```python
from build123d import *

# Parameters (mm, degrees)
SKETCH3_R           = 27.045923136
BOSS_EXTRUDE1_DEPTH = 5.6
SKETCH4_R           = 1.5
CUT_EXTRUDE1_DEPTH  = 6.6
BOSS_EXTRUDE3_DEPTH = 5.6
SKETCH6_R           = 4.2
BOSS_EXTRUDE4_DEPTH = 8.4
SKETCH7_W           = 5.4
SKETCH7_H           = 3.76
CUT_EXTRUDE2_DEPTH  = 6
FILLET1_R           = 4


with BuildPart() as part:
    # Sketch3 → Boss-Extrude1 (new body)
    with BuildSketch(Plane(origin=(0, 0, 0), x_dir=(0, 0, -1), z_dir=(1, 0, 0))):
        Circle(SKETCH3_R)
    extrude(amount=BOSS_EXTRUDE1_DEPTH)

    # Sketch4 → Cut-Extrude1 (cut, through all)
    with BuildSketch(Plane(origin=(5.6, 0, 0), x_dir=(0, 0, -1), z_dir=(1, 0, 0))):
        with Locations((0, 27.045923136)):
            Circle(SKETCH4_R)
        with Locations((13.522961568, 23.422456505)):
            Circle(SKETCH4_R)
        with Locations((23.422456505, 13.522961568)):
            Circle(SKETCH4_R)
        with Locations((27.045923136, 0)):
            Circle(SKETCH4_R)
        with Locations((23.422456505, -13.522961568)):
            Circle(SKETCH4_R)
        with Locations((13.522961568, -23.422456505)):
            Circle(SKETCH4_R)
        with Locations((0, -27.045923136)):
            Circle(SKETCH4_R)
        with Locations((-13.522961568, -23.422456505)):
            Circle(SKETCH4_R)
        with Locations((-23.422456505, -13.522961568)):
            Circle(SKETCH4_R)
        with Locations((-27.045923136, 0)):
            Circle(SKETCH4_R)
        with Locations((-23.422456505, 13.522961568)):
            Circle(SKETCH4_R)
        with Locations((-13.522961568, 23.422456505)):
            Circle(SKETCH4_R)
    extrude(amount=-CUT_EXTRUDE1_DEPTH, mode=Mode.SUBTRACT)

    # Sketch5 → Boss-Extrude3 (add)
    with BuildSketch(Plane(origin=(5.6, 0, 0), x_dir=(0, 0, -1), z_dir=(1, 0, 0))):
        with BuildLine():
            Line((1.499423149, 27.004327218), (4.76164368, 32.654658924))
            ThreePointArc((4.76164368, 32.654658924), (8.541028488, 31.875552268), (12.203625071, 30.660586021))
            Line((12.203625071, 30.660586021), (12.203625071, 24.136144957))
            Line((12.203625071, 24.136144957), (2.679491924, 10))
            Line((2.679491924, 10), (1.499423149, 27.004327218))
        make_face()
        with BuildLine():
            Line((22.636721809, 14.800702147), (7.320508076, 7.320508076))
            Line((7.320508076, 7.320508076), (14.800702147, 22.636721809))
            Line((14.800702147, 22.636721809), (20.451033853, 25.89894234))
            ThreePointArc((20.451033853, 25.89894234), (23.334523779, 23.334523779), (25.89894234, 20.451033853))
            Line((25.89894234, 20.451033853), (22.636721809, 14.800702147))
        make_face()
        with BuildLine():
            Line((27.004327218, 1.499423149), (10, 2.679491924))
            Line((10, 2.679491924), (24.136144957, 12.203625071))
            Line((24.136144957, 12.203625071), (30.660586021, 12.203625071))
            ThreePointArc((30.660586021, 12.203625071), (31.875552268, 8.541028488), (32.654658924, 4.76164368))
            Line((32.654658924, 4.76164368), (27.004327218, 1.499423149))
        make_face()
        with BuildLine():
            Line((24.136144957, -12.203625071), (10, -2.679491924))
            Line((10, -2.679491924), (27.004327218, -1.499423149))
            Line((27.004327218, -1.499423149), (32.654658924, -4.76164368))
            ThreePointArc((32.654658924, -4.76164368), (31.875552268, -8.541028488), (30.660586021, -12.203625071))
            Line((30.660586021, -12.203625071), (24.136144957, -12.203625071))
        make_face()
        with BuildLine():
            Line((14.800702147, -22.636721809), (7.320508076, -7.320508076))
            Line((7.320508076, -7.320508076), (22.636721809, -14.800702147))
            Line((22.636721809, -14.800702147), (25.89894234, -20.451033853))
            ThreePointArc((25.89894234, -20.451033853), (23.334523779, -23.334523779), (20.451033853, -25.89894234))
            Line((20.451033853, -25.89894234), (14.800702147, -22.636721809))
        make_face()
        with BuildLine():
            Line((1.499423149, -27.004327218), (2.679491924, -10))
            Line((2.679491924, -10), (12.203625071, -24.136144957))
            Line((12.203625071, -24.136144957), (12.203625071, -30.660586021))
            ThreePointArc((12.203625071, -30.660586021), (8.541028488, -31.875552268), (4.76164368, -32.654658924))
            Line((4.76164368, -32.654658924), (1.499423149, -27.004327218))
        make_face()
        with BuildLine():
            Line((-12.203625071, -24.136144957), (-2.679491924, -10))
            Line((-2.679491924, -10), (-1.499423149, -27.004327218))
            Line((-1.499423149, -27.004327218), (-4.76164368, -32.654658924))
            ThreePointArc((-4.76164368, -32.654658924), (-8.541028488, -31.875552268), (-12.203625071, -30.660586021))
            Line((-12.203625071, -30.660586021), (-12.203625071, -24.136144957))
        make_face()
        with BuildLine():
            Line((-22.636721809, -14.800702147), (-7.320508076, -7.320508076))
            Line((-7.320508076, -7.320508076), (-14.800702147, -22.636721809))
            Line((-14.800702147, -22.636721809), (-20.451033853, -25.89894234))
            ThreePointArc((-20.451033853, -25.89894234), (-23.334523779, -23.334523779), (-25.89894234, -20.451033853))
            Line((-25.89894234, -20.451033853), (-22.636721809, -14.800702147))
        make_face()
        with BuildLine():
            Line((-27.004327218, -1.499423149), (-10, -2.679491924))
            Line((-10, -2.679491924), (-24.136144957, -12.203625071))
            Line((-24.136144957, -12.203625071), (-30.660586021, -12.203625071))
            ThreePointArc((-30.660586021, -12.203625071), (-31.875552268, -8.541028488), (-32.654658924, -4.76164368))
            Line((-32.654658924, -4.76164368), (-27.004327218, -1.499423149))
        make_face()
        with BuildLine():
            Line((-24.136144957, 12.203625071), (-10, 2.679491924))
            Line((-10, 2.679491924), (-27.004327218, 1.499423149))
            Line((-27.004327218, 1.499423149), (-32.654658924, 4.76164368))
            ThreePointArc((-32.654658924, 4.76164368), (-31.875552268, 8.541028488), (-30.660586021, 12.203625071))
            Line((-30.660586021, 12.203625071), (-24.136144957, 12.203625071))
        make_face()
        with BuildLine():
            Line((-14.800702147, 22.636721809), (-7.320508076, 7.320508076))
            Line((-7.320508076, 7.320508076), (-22.636721809, 14.800702147))
            Line((-22.636721809, 14.800702147), (-25.89894234, 20.451033853))
            ThreePointArc((-25.89894234, 20.451033853), (-23.334523779, 23.334523779), (-20.451033853, 25.89894234))
            Line((-20.451033853, 25.89894234), (-14.800702147, 22.636721809))
        make_face()
        with BuildLine():
            Line((-1.499423149, 27.004327218), (-2.679491924, 10))
            Line((-2.679491924, 10), (-12.203625071, 24.136144957))
            Line((-12.203625071, 24.136144957), (-12.203625071, 30.660586021))
            ThreePointArc((-12.203625071, 30.660586021), (-8.541028488, 31.875552268), (-4.76164368, 32.654658924))
            Line((-4.76164368, 32.654658924), (-1.499423149, 27.004327218))
        make_face()
    extrude(amount=-BOSS_EXTRUDE3_DEPTH)

    # Sketch6 → Boss-Extrude4 (add)
    with BuildSketch(Plane(origin=(5.6, 0, 0), x_dir=(0, 0, -1), z_dir=(1, 0, 0))):
        Circle(SKETCH6_R)
    extrude(amount=BOSS_EXTRUDE4_DEPTH)

    # Sketch7 → Cut-Extrude2 (cut)
    with BuildSketch(Plane(origin=(14, 0, 0), x_dir=(0, 0, -1), z_dir=(1, 0, 0))):
        Rectangle(SKETCH7_W, SKETCH7_H)
    extrude(amount=-CUT_EXTRUDE2_DEPTH, mode=Mode.SUBTRACT)

    # Fillet1
    fillet1_edges = [part.edges().sort_by_distance(p)[0] for p in [
        (5.6, 0, 4.2),
    ]]
    fillet(fillet1_edges, radius=FILLET1_R)


solid = part.part
```
Model file for the job. Use its own axes, mm. A direction names the side the tool comes from. Coordinates: 2 decimals unless noted, no trailing zeros. Order: outer loops, then holes, each group sorted by start corner. A loop starts at its lowest first (then second) coordinate and runs counter-clockwise, first axis right, second up. Notation, with made-up numbers: (42, -25) - (98, -25) arc R35 ccw to (98, 8) - close; hole circle Ø9 at (-16.5, 9). An arc over 180 degrees is marked (long way). Return JSON: item names as keys, results as strings. Group by question number.
1) Tool access for faces 1 (the flat face through (3, 12.204, -27)), 2 (the flat face through (2.839, -24.245, 17.586)), 3 (the flat face through (2.84, 29.79, -3.11)), 4 (the flat face through (3, -12.204, 27)), 5 (the flat face through (5.6, -7, 7)): list every direction of +Z, -Z, +X, -X, +Y, -Y with a clear straight run to the whole face (end or side of a thin tool).
2) Mould opens along Y. For faces 6 (the cylindrical face through (2.839, 12.745, 22.14)), 7 (the cylindrical face through (2.839, -12.745, -22.14)), 8 (the cylindrical face through (2.839, -8.593, 31.862)), 9 (the flat face through (2.839, 24.245, -17.586)) say: released by +Y, released by -Y, zero draft, split by the parting line, or undercut.
3) Saw through at A-A, the plane x = 10.75. Write the cut outline in (y, z), plus the area to 3 significant figures.
4) Saw through at C-C, the plane y = 0. Write the cut outline in (x, z).
5) Probe line 1 (Y direction, x = 0.5, z = -27); line 2 (X direction, y = 9, z = 2.5); line 3 (X direction, y = 6, z = -4.5). List the from-to ranges inside material, lowest first. Write a range as from..to.
6) Flat gauge pins, fed straight in: P1, Ø1, axis at x = 11.5, z = 0, coming from the +Y side; P2, Ø1, axis at y = -15, z = 19, coming from the +X side; P3, Ø3, axis at x = 3.5, z = 27, coming from the +Y side; P4, Ø8, axis at x = 5.5, z = -8.5, coming from the +Y side. Where does each tip first touch, or does it go through?
7) Saw through at D-D, the plane x = 6.5. Write the cut outline in (y, z), plus the area to 3 significant figures.
8) Saw through at B-B, the plane z = 0. Write the cut outline in (x, y), plus the area to 3 significant figures.
Values found:
{
 "1": {"face 1": "-Z, +X, -X", "face 2": "+X, -X, -Y", "face 3": "+X, -X, +Y", "face 4": "+Z, +X, -X", "face 5": "+X"},
 "2": {"face 6": "undercut", "face 7": "undercut", "face 8": "released by -Y", "face 9": "released by +Y"},
 "3": {"outline": "circle Ø8.4 at (0, 0); hole (-1.88, -2.7) - (1.88, -2.7) - (1.88, 2.7) - (-1.88, 2.7) - close", "area": "35.1 mm²"},
 "4": {"outline": "(0, -25.55) - (5.6, -25.55) - (5.6, -8.2) arc R4 cw to (9.6, -4.2) - (14, -4.2) - (14, -2.7) - (8, -2.7) - (8, 2.7) - (14, 2.7) - (14, 4.2) - (9.6, 4.2) arc R4 cw to (5.6, 8.2) - (5.6, 25.55) - (0, 25.55) - close"},
 "5": {"line 1": "y = -12.2..-1.5, 1.5..12.2", "line 2": "x = 0..5.6", "line 3": "x = 0..5.66"},
 "6": {"P1": "stops at y = 4.2", "P2": "stops at x = 5.6", "P3": "stops at y = 20.95", "P4": "stops at y = 32.65"},
 "7": {"outline": "circle Ø11.34 at (0, 0)", "area": "101 mm²"},
 "8": {"outline": "(0, -25.55) - (5.6, -25.55) - (5.6, -8.2) arc R4 cw to (9.6, -4.2) - (14, -4.2) - (14, -1.88) - (8, -1.88) - (8, 1.88) - (14, 1.88) - (14, 4.2) - (9.6, 4.2) arc R4 cw to (5.6, 8.2) - (5.6, 25.55) - (0, 25.55) - close", "area": "341 mm²"}
}
